from build123d import *

# Parameters (mm, degrees)
BOSS_EXTRUDE1_DEPTH = 20
SKETCH2_W           = 55.254397281
SKETCH2_H           = 28.618836095
BOSS_EXTRUDE5_DEPTH = 30
SKETCH3_R           = 11.008857327
SKETCH3_W           = 54.887017246
SKETCH3_H           = 22.017714654
CUT_EXTRUDE1_DEPTH  = 30


with BuildPart() as part:
    # Sketch1 → Boss-Extrude1 (new body)
    with BuildSketch(Plane(origin=(0, 0, 0), x_dir=(1, 0, 0), z_dir=(0, 1, 0))):
        with BuildLine():
            Line((-75, 50), (75, 50))
            ThreePointArc((75, 50), (125, 0), (75, -50))
            Line((75, -50), (-75, -50))
            Line((-75, -50), (-75, 50))
        make_face()
    extrude(amount=BOSS_EXTRUDE1_DEPTH)

    # Sketch2 → Boss-Extrude5 (add)
    with BuildSketch(Plane(origin=(0, 20, 0), x_dir=(1, 0, 0), z_dir=(0, 1, 0))):
        with Locations((-47.37280136, -35.690581952)):
            Rectangle(SKETCH2_W, SKETCH2_H)
    extrude(amount=BOSS_EXTRUDE5_DEPTH)

    # Sketch3 → Cut-Extrude1 (cut)
    with BuildSketch(Plane(origin=(0, 20, 0), x_dir=(1, 0, 0), z_dir=(0, 1, 0))):
        with Locations((27.443508623, 0)):
            Circle(SKETCH3_R)
        Rectangle(SKETCH3_W, SKETCH3_H)
    extrude(amount=-CUT_EXTRUDE1_DEPTH, mode=Mode.SUBTRACT)


solid = part.part
Work out the finished part from the listing and answer in its coordinate system (mm). A direction names the side the tool comes from. Coordinates: 2 decimals unless noted, no trailing zeros. Write each loop counter-clockwise with the first axis right and the second up, starting at its lowest first coordinate (ties: lowest second). Pieces come first, ordered by that corner, then holes.
1. Consider line 1 along Y through (x, z) = (-28, -29); line 2 along Z through (x, y) = (-27, 21.5); line 3 along Z through (x, y) = (-8.5, 6.5). Determine where each line is inside the solid, lowest interval first.
Results list:
line 1: y = 0 to 20
line 2: z = 21.38 to 50
line 3: z = -50 to -11.01, 11.01 to 50
2. The part is cut by section B-B, the plane z = 0. Write down the section's boundary in (x, y), and give its area (3 significant figures).
Results list:
outline: (-75, 0) - (-27.44, 0) - (-27.44, 20) - (-75, 20) - close; (38.45, 0) - (125, 0) - (125, 20) - (38.45, 20) - close
area: 2,680 mm2
3. The part is cut by section D-D, the plane x = -40.5. Write down the section's boundary in (y, z).
Results list:
outline: (0, -50) - (20, -50) - (20, 21.38) - (50, 21.38) - (50, 50) - (0, 50) - close
4. For faces 1 (the cylindrical face through (38.45, 10.14, 0.24)), 2 (the flat face through (-1, 10, -50)), 3 (the flat face through (-48, 35, 21.381)), 4 (the flat face through (-19.746, 35, 36)), 5 (the flat face through (-75, 19, 12)), determine the directions among +Z, -Z, +X, -X, +Y, -Y from which every point of the face is accessible in a straight line to the end or side of a thin tool.
Results list:
face 1: +Y, -Y
face 2: -Z, +X, -X, +Y, -Y
face 3: -Z, +X, -X, +Y
face 4: +Z, -Z, +X, +Y
face 5: +Z, -Z, -X, +Y, -Y
5. For a pull along Z with two mould halves and no side action, classify faces 6 (the cylindrical face through (124.988, 9.86, -1.099)), 7 (the flat face through (-27.444, 10, 0)), 8 (the flat face through (0, 10, -11.009)), 9 (the flat face through (-48, 50, 35)) as +Z half, -Z half, draft (parallel to the pull), parting line (faces both ways), or undercut.
Results list:
face 6: parting line
face 7: undercut
face 8: undercut
face 9: draft
6. The part is cut by section C-C, the plane y = 12.5. Write down the section's boundary in (x, z), and give its area (3 significant figures).
Results list:
outline: (-75, -50) - (75, -50) arc R50 ccw to (75, 50) - (-75, 50) - close; hole (-27.44, -11.01) - (27.44, -11.01) arc R11.01 ccw to (27.44, 11.01) - (-27.44, 11.01) - close
area: 17,500 mm2
7. Flat-ended cylindrical pins translate along their axes: pin 1 (1 mm diameter, centred on x = 63.5, z = -31.5, fed in from +Y); pin 2 (15 mm diameter, centred on x = -40, y = 41.5, fed in from -Z); pin 3 (6 mm diameter, centred on y = 7, z = -2.5, fed in from +X). Find the tip coordinate at first contact, or state that the pin passes through.
Results list:
pin 1: stops at y = 20
pin 2: stops at z = 21.38
pin 3: stops at x = 125
8. The part is cut by section A-A, the plane x = 5. Write down the section's boundary in (y, z).
Results list:
outline: (0, -50) - (20, -50) - (20, -11.01) - (0, -11.01) - close; (0, 11.01) - (20, 11.01) - (20, 50) - (0, 50) - close
